Read the model definition and answer for the solid it produces. Units are mm, in the model's axes. A direction names the side the tool comes from. Coordinates: 2 decimals unless noted, no trailing zeros. Loops run counter-clockwise (first coordinate to the right, second up) from the corner with the lowest first, then second, coordinate; pieces in that order, holes last.
from build123d import *
from build123d.topology import SkipClean

# Parameters (mm, degrees)
BOSS_EXTRUDE1_START           = 5
BOSS_EXTRUDE1_DEPTH           = 6
CHAMFER1_SIZE                 = 4.5
SKETCH2_W                     = 6
SKETCH2_H                     = 6.3
BOSS_EXTRUDE2_DEPTH           = 6.3
BOSS_EXTRUDE3_DEPTH           = 7.3
BOSS_EXTRUDE4_DEPTH           = 14.405295
CSK_FOR_M3_SFHCS1_D           = 3
CSK_FOR_M3_SFHCS1_CSINK_D     = 6.3
CSK_FOR_M3_SFHCS1_CSINK_ANGLE = 90
BOSS_EXTRUDE5_DEPTH           = 14.405295
CSK_FOR_M3_SFHCS2_D           = 3
CSK_FOR_M3_SFHCS2_CSINK_D     = 6.3
CSK_FOR_M3_SFHCS2_CSINK_ANGLE = 90
SKETCH10_W                    = 19.443915682
SKETCH10_H                    = 19.443915683
CUT_EXTRUDE1_DEPTH            = 15
CSK_FOR_M3_SFHCS3_D           = 3
CSK_FOR_M3_SFHCS3_DEPTH       = 96.77876722
CSK_FOR_M3_SFHCS3_CSINK_D     = 6.3
CSK_FOR_M3_SFHCS3_CSINK_ANGLE = 90


with BuildPart() as part:
    # Sketch1 → Boss-Extrude1 (new body)
    with BuildSketch(Plane.XY.offset(BOSS_EXTRUDE1_START)):
        with BuildLine():
            Line((-23.5, -12), (-7, -12))
            Line((-7, -12), (-7, -8.5))
            ThreePointArc((-7, -8.5), (-6.853553391, -8.146446609), (-6.5, -8))
            Line((-6.5, -8), (6.5, -8))
            ThreePointArc((6.5, -8), (6.853553391, -8.146446609), (7, -8.5))
            Line((7, -8.5), (7, -12))
            Line((7, -12), (23.5, -12))
            Line((23.5, -12), (26, -9.5))
            Line((26, -9.5), (26, -3.15))
            Line((26, -3.15), (32.3, -3.15))
            Line((32.3, -3.15), (32.3, 3.15))
            Line((32.3, 3.15), (26, 3.15))
            Line((26, 3.15), (26, 9.5))
            Line((26, 9.5), (23.5, 12))
            Line((23.5, 12), (6, 12))
            Line((6, 12), (6, 5.5))
            ThreePointArc((6, 5.5), (5.853553391, 5.146446609), (5.5, 5))
            Line((5.5, 5), (-5.5, 5))
            ThreePointArc((-5.5, 5), (-5.853553391, 5.146446609), (-6, 5.5))
            Line((-6, 5.5), (-6, 12))
            Line((-6, 12), (-23.5, 12))
            Line((-23.5, 12), (-26, 9.5))
            Line((-26, 9.5), (-26, 3.15))
            Line((-26, 3.15), (-32.3, 3.15))
            Line((-32.3, 3.15), (-32.3, -3.15))
            Line((-32.3, -3.15), (-26, -3.15))
            Line((-26, -3.15), (-26, -9.5))
            Line((-26, -9.5), (-23.5, -12))
        make_face()
    extrude(amount=BOSS_EXTRUDE1_DEPTH)

    # Chamfer1
    chamfer1_edges = [part.edges().sort_by_distance(p)[0] for p in [
        (7, -10.25, 5),
        (6.853553391, -8.146446609, 5),
        (0, -8, 5),
        (-6.853553391, -8.146446609, 5),
        (-7, -10.25, 5),
    ]]
    chamfer(chamfer1_edges, length=CHAMFER1_SIZE)

    # Sketch2 → Boss-Extrude2 (add)
    with BuildSketch(Plane(origin=(26, 0, 0), x_dir=(0, 0, -1), z_dir=(1, 0, 0))):
        with Locations((-8, 0)):
            Rectangle(SKETCH2_W, SKETCH2_H)
    boss_extrude2 = extrude(amount=BOSS_EXTRUDE2_DEPTH)

    # Mirror1: Boss-Extrude2 across plane
    add(boss_extrude2.mirror(Plane(origin=(0, 0, 0), x_dir=(0, 0, 1), z_dir=(1, 0, 0))))

    # Sketch3 → Boss-Extrude3 (add)
    with BuildSketch(Plane.XY.offset(11)):
        Polygon((11.551404138, 1.816830905), (2.291859281, -9.218264944), (8.439052056, -14.376372134), (17.698596913, -3.341276285), align=None)
    boss_extrude3 = extrude(amount=BOSS_EXTRUDE3_DEPTH)

    # Sketch4 → Boss-Extrude4 (add)
    with SkipClean():  # the faces are left unmerged after this step: merging them gives an invalid solid
        with BuildSketch(Plane(origin=(5.667376511, 6.754116317, 0), x_dir=(0.7660444431189792, -0.6427876096865379, 0), z_dir=(0.6427876096865379, 0.7660444431189792, 0))):
            with BuildLine():
                Line((15.705642813, -18.3), (7.681052555, -18.3))
                ThreePointArc((7.681052555, -18.3), (11.693347684, -22.312295129), (15.705642813, -18.3))
            make_face()
        extrude(amount=-BOSS_EXTRUDE4_DEPTH)

    # CSK for M3 SFHCS1 (through all)
    with Locations(Plane(origin=(5.667376511, 6.754116317, 0), x_dir=(0.7660444431189792, -0.6427876096865379, 0), z_dir=(0.6427876096865379, 0.7660444431189792, 0))):
        with Locations((11.693347684, -18.3)):
            CounterSinkHole(CSK_FOR_M3_SFHCS1_D / 2, CSK_FOR_M3_SFHCS1_CSINK_D / 2, counter_sink_angle=CSK_FOR_M3_SFHCS1_CSINK_ANGLE)

    # Mirror11: Boss-Extrude3 across plane
    with SkipClean():  # the faces are left unmerged after this step: merging them gives an invalid solid
        add(boss_extrude3.mirror(Plane(origin=(0, 0, 0), x_dir=(0, 0, 1), z_dir=(1, 0, 0))))

    # Sketch7 → Boss-Extrude5 (add)
    with SkipClean():  # the faces are left unmerged after this step: merging them gives an invalid solid
        with BuildSketch(Plane(origin=(-5.667376511, 6.754116317, 0), x_dir=(0.7660444431189792, 0.6427876096865379, 0), z_dir=(-0.6427876096865379, 0.7660444431189792, 0))):
            with BuildLine():
                Line((-15.705642813, -18.3), (-7.681052555, -18.3))
                ThreePointArc((-7.681052555, -18.3), (-11.693347684, -22.312295129), (-15.705642813, -18.3))
            make_face()
        extrude(amount=-BOSS_EXTRUDE5_DEPTH)

    # CSK for M3 SFHCS2 (through all)
    with Locations(Plane(origin=(-5.667376511, 6.754116317, 0), x_dir=(0.7660444431189792, 0.6427876096865379, 0), z_dir=(-0.6427876096865379, 0.7660444431189792, 0))):
        with Locations((-11.693347684, -18.3)):
            CounterSinkHole(CSK_FOR_M3_SFHCS2_D / 2, CSK_FOR_M3_SFHCS2_CSINK_D / 2, counter_sink_angle=CSK_FOR_M3_SFHCS2_CSINK_ANGLE)

    # Sketch10 → Cut-Extrude1 (cut)
    with SkipClean():  # the faces are left unmerged after this step: merging them gives an invalid solid
        with BuildSketch(Plane.XY.offset(11)):
            with Locations((9.721957841, -5.898825434)):
                Rectangle(SKETCH10_W, SKETCH10_H)
        extrude(amount=CUT_EXTRUDE1_DEPTH, mode=Mode.SUBTRACT)

    # CSK for M3 SFHCS3
    with Locations(Plane(origin=(1373.834887972, -105.616816862, -567.783106147), x_dir=(0.6343091461006831, 0.5322485705454647, -0.5606811628058603), z_dir=(0.4295066891289175, 0.36039890443624706, 0.8280317830099689))):
        with Locations((-1114.335057549, 945.253960578), (-1158.995448583, 982.728478223)):
            CounterSinkHole(CSK_FOR_M3_SFHCS3_D / 2, CSK_FOR_M3_SFHCS3_CSINK_D / 2, depth=CSK_FOR_M3_SFHCS3_DEPTH, counter_sink_angle=CSK_FOR_M3_SFHCS3_CSINK_ANGLE)


solid = part.part
Item 1: Which of the six approach directions +Z, -Z, +X, -X, +Y, -Y give full straight-line access (tool end or side, diameter ignored) to faces 4 (the face through (0, 5, 8)), 5 (the face through (-28, -3.15, 8)), 6 (the face through (8.445, -6.512, 7.218))?
Numbers:
face 4: +Z, -Z, +Y
face 5: +Z, -Z, -X, -Y
face 6: -Z, -Y
Item 2: Find the intervals of material crossed by line 1 along Z through (x, y) = (11.5, -5); line 2 along Y through (x, z) = (-5, 8.5); line 3 along X through (y, z) = (-11.25, 8.25), in increasing order.
Numbers:
line 1: z = 5 to 11
line 2: y = -7 to 5
line 3: x = -24.25 to -8.25, 8.25 to 24.25
Item 3: A cutting plane is placed at B-B on y = 4. Determine the outline of the cut face in (x, z).
Numbers:
outline: (-26, 5) - (26, 5) - (26, 11) - (-26, 11) - close
Item 4: Given pin 1 (5 mm diameter, centred on y = -6.5, z = 9, fed in from -X); pin 2 (8 mm diameter, centred on x = 24.5, z = 7.5, fed in from -Y); pin 3 (2 mm diameter, centred on x = -15, z = 13.5, fed in from -Y); pin 4 (5 mm diameter, centred on x = 16.5, z = 15.5, fed in from -Y), each flat-ended and moving along its own axis, determine where each tip first touches the part or whether it passes through.
Numbers:
pin 1: stops at x = -26
pin 2: stops at y = -12
pin 3: stops at y = -7.75
pin 4: passes through
Item 5: A cutting plane is placed at A-A on x = -1. Determine the outline of the cut face in (y, z).
Numbers:
outline: (-8, 9.5) - (-3.5, 5) - (5, 5) - (5, 11) - (-8, 11) - close
Item 6: Determine the mould class of faces 1 (the face through (26, -6, 8)), 2 (the face through (31.547, 2.133, 6.084)), 3 (the face through (-0.1, -5.7, 7.2)) for opening direction Y: released by +Y, released by -Y, zero draft, split by the parting line, or undercut.
Numbers:
face 1: zero draft
face 2: undercut
face 3: released by -Y
Item 7: A cutting plane is placed at C-C on z = 13.75. Determine the outline of the cut face in (x, y).
Numbers:
outline: (-17.7, -3.34) - (-8.44, -14.38) - (-2.29, -9.22) - (-11.55, 1.82) - close
